```python
from build123d import *

# Parameters (mm, degrees)
SKETCH1_W           = 78
SKETCH1_H           = 96
BOSS_EXTRUDE1_DEPTH = 3
SKETCH2_R           = 2.5
CUT_EXTRUDE1_DEPTH  = 3
SKETCH3_W           = 48
SKETCH3_H           = 36.000458934
CUT_EXTRUDE2_DEPTH  = 3


with BuildPart() as part:
    # Sketch1 → Boss-Extrude1 (new body)
    with BuildSketch(Plane(origin=(0, 0, 0), x_dir=(1, 0, 0), z_dir=(0, 1, 0))):
        with Locations((39, 48)):
            Rectangle(SKETCH1_W, SKETCH1_H)
    extrude(amount=BOSS_EXTRUDE1_DEPTH)

    # Sketch2 → Cut-Extrude1 (cut)
    with BuildSketch(Plane(origin=(0, 3, 0), x_dir=(1, 0, 0), z_dir=(0, 1, 0))):
        with Locations(Location((8, 6, 0), (0, 0, 270))):
            Circle(SKETCH2_R)
        with Locations(Location((26, 6, 0), (0, 0, 270))):
            Circle(SKETCH2_R)
        with Locations(Location((8, 24, 0), (0, 0, 270))):
            Circle(SKETCH2_R)
        with Locations(Location((26, 24, 0), (0, 0, 270))):
            Circle(SKETCH2_R)
        with Locations(Location((52, 6, 0), (0, 0, 270))):
            Circle(SKETCH2_R)
        with Locations(Location((70, 6, 0), (0, 0, 270))):
            Circle(SKETCH2_R)
        with Locations(Location((70, 24, 0), (0, 0, 270))):
            Circle(SKETCH2_R)
        with Locations(Location((52, 24, 0), (0, 0, 270))):
            Circle(SKETCH2_R)
        with Locations(Location((48.001269273, 72.000000045, 0), (0, 0, 270))):
            Circle(SKETCH2_R)
        with Locations(Location((30.001269279, 72.000458934, 0), (0, 0, 270))):
            Circle(SKETCH2_R)
        with Locations(Location((48, 90, 0), (0, 0, 270))):
            Circle(SKETCH2_R)
        with Locations(Location((30.000000006, 90.000458889, 0), (0, 0, 270))):
            Circle(SKETCH2_R)
    extrude(amount=-CUT_EXTRUDE1_DEPTH, mode=Mode.SUBTRACT)

    # Sketch3 → Cut-Extrude2 (cut)
    with BuildSketch(Plane(origin=(0, 3, 0), x_dir=(1, 0, 0), z_dir=(0, 1, 0))):
        with Locations((39, 48.000229467)):
            Rectangle(SKETCH3_W, SKETCH3_H)
    extrude(amount=-CUT_EXTRUDE2_DEPTH, mode=Mode.SUBTRACT)


solid = part.part
```
Part model, mm, in its own coordinate system. A direction names the side the tool comes from. Round coordinates to 2 decimals unless told otherwise and drop trailing zeros. Write each loop counter-clockwise with the first axis right and the second up, starting at its lowest first coordinate (ties: lowest second). Pieces come first, ordered by that corner, then holes.
Item 1: Drop a flat-ended pin along its axis: pin 1 Ø6.5 at (x, z) = (52, -6) entering from +Y. Give the stop position or say it passes through.
Results:
pin 1: stops at y = 3
Item 2: Which spindle directions (+Z, -Z, +X, -X, +Y, -Y) get a long thin tool onto all of the face, cutting with end or side? Do faces 1 (the flat face through (63, 2, -48)), 2 (the flat face through (0, 1, -47)). Say none if no direction does.
Results:
face 1: +Y, -Y
face 2: +Z, -Z, -X, +Y, -Y
Item 3: Two-plate mould, pull along Z, no slides. Class faces 3 (the cylindrical face through (67.78, 1.52, -4.85)), 4 (the flat face through (38, 1, -96)), 5 (the flat face through (78, 1, -47)): +Z half, -Z half, draft (parallel to the pull), parting line (faces both ways), or undercut.
Results:
face 3: undercut
face 4: -Z half
face 5: draft
Item 4: Cut at C-C, the plane x = 57. Give the cut face in (y, z).
Results:
outline: (0, -96) - (3, -96) - (3, -66) - (0, -66) - close; (0, -30) - (3, -30) - (3, 0) - (0, 0) - close
Item 5: Cut at B-B, the plane z = -24. Give the cut face in (x, y).
Results:
outline: (0, 0) - (5.5, 0) - (5.5, 3) - (0, 3) - close; (10.5, 0) - (23.5, 0) - (23.5, 3) - (10.5, 3) - close; (28.5, 0) - (49.5, 0) - (49.5, 3) - (28.5, 3) - close; (54.5, 0) - (67.5, 0) - (67.5, 3) - (54.5, 3) - close; (72.5, 0) - (78, 0) - (78, 3) - (72.5, 3) - close
Item 6: Cut at D-D, the plane x = 8. Give the cut face in (y, z), plus the area to 3 significant figures.
Results:
outline: (0, -96) - (3, -96) - (3, -26.5) - (0, -26.5) - close; (0, -21.5) - (3, -21.5) - (3, -8.5) - (0, -8.5) - close; (0, -3.5) - (3, -3.5) - (3, 0) - (0, 0) - close
area: 258 mm2
Item 7: Cut at A-A, the plane z = -58.5. Give the cut face in (x, y).
Results:
outline: (0, 0) - (15, 0) - (15, 3) - (0, 3) - close; (63, 0) - (78, 0) - (78, 3) - (63, 3) - close
Item 8: Probe L1, parallel to X at y = 0.75, z = -24; L2, parallel to X at y = 0.6, z = -63; L3, parallel to Z at x = 9.5, y = 0.55. List the from-to ranges inside material, lowest first.
Results:
L1: x = 0 to 5.5, 10.5 to 23.5, 28.5 to 49.5, 54.5 to 67.5, 72.5 to 78
L2: x = 0 to 15, 63 to 78
L3: z = -96 to -26, -22 to -8, -4 to 0
